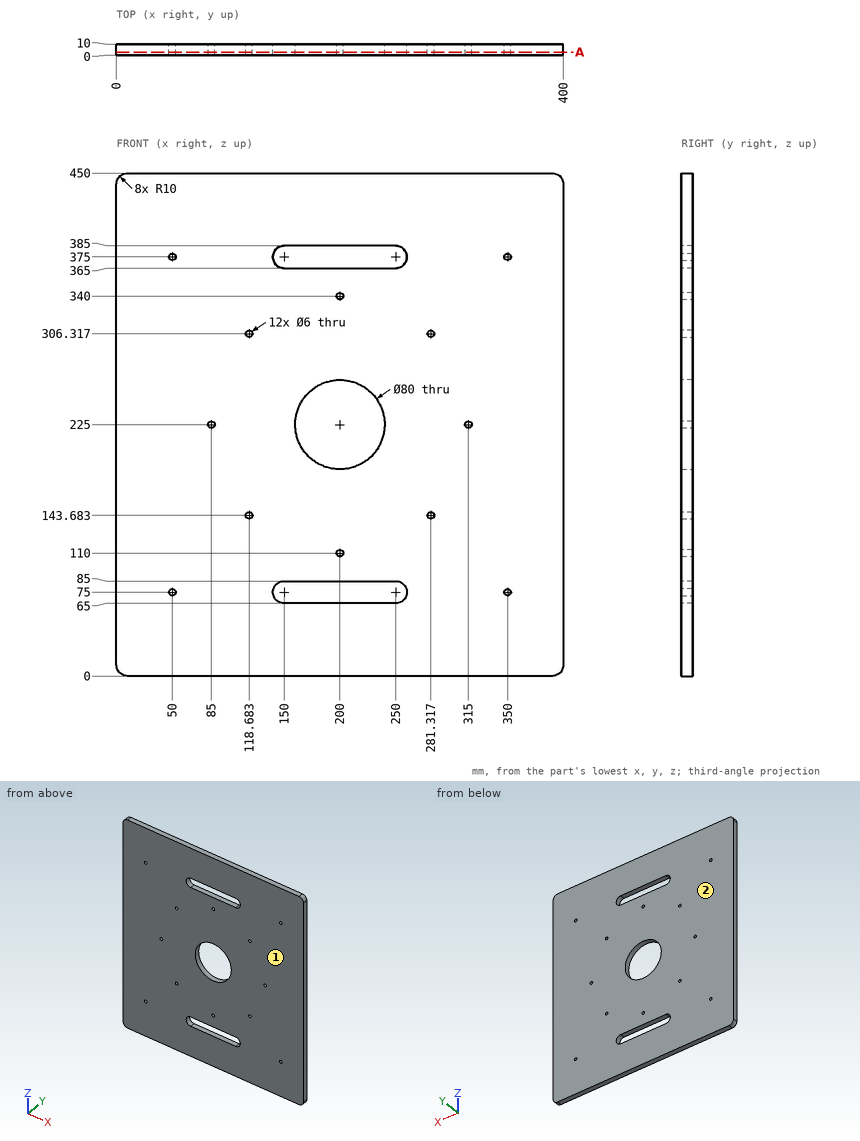
Input: dimensioned drawing with shaded views. Units: mm. Origin: part minimum x, y, z. Give positions to 0.01 mm unless a question says otherwise; leave off trailing zeros. Return JSON: item names as keys, results as strings. Group by question number.
1. Material intervals for line 1 (X direction, y = 2.25, z = 225); line 2 (X direction, y = 5.25, z = 75); line 3 (Z direction, x = 85, y = 4.75), sorted ascending. Write a range as from..to.
2. Section A-A, the plane y = 2.75. Count the separate pieces of the cut face and the enclosed holes in it, then the cut area to 3 significant figures.
3. Mould query, pull axis Y, two halves, no side actions, for the marked faces 1 and 2. Classes: +Y half, -Y half, draft (parallel to the pull), parting line (faces both ways), or undercut.
Determined:
{
 "1": {"line 1": "x = 0..82, 88..160, 240..312, 318..400", "line 2": "x = 0..47, 53..140, 260..347, 353..400", "line 3": "z = 0..222, 228..450"},
 "2": {"separate pieces": "1", "enclosed holes": "15", "area": "170,000 mm2"},
 "3": {"face 1": "-Y half", "face 2": "+Y half"}
}
